from build123d import *

# Parameters (mm, degrees)
EXTRUDE_1_DEPTH          = 22
PATTERN_LINEAR_1_COUNT   = 2
PATTERN_LINEAR_1_PITCH   = 23.5
CUT_EXTRUDE_1_DEPTH      = 38.269290307
CUT_EXTRUDE_1_DEPTH_BACK = 38.269290307
SKETCH_4_W               = 15.894607506
SKETCH_4_H               = 11.25
SKETCH_4_W_2             = 16.409425433
SKETCH_4_H_2             = 14.25
SKETCH_5_R               = 2.5
CUT_EXTRUDE_2_DEPTH      = 45.469793118


with BuildPart() as part:
    # 草图1 → 凸台-拉伸1 (new, symmetric)
    with BuildSketch(Plane.XY):
        with BuildLine():
            Line((29, -5.5), (29, -8))
            Line((29, -8), (1, -8))
            Line((1, -8), (-1.370141735, -7.373785434))
            ThreePointArc((-1.370141735, -7.373785434), (-4.794472702, 5.767411162), (7.5, 0))
            Line((7.5, 0), (25.406366901, 0))
            ThreePointArc((25.406366901, 0), (25.916831332, -0.140101131), (26.284262474, -0.521147869))
            Line((26.284262474, -0.521147869), (29, -5.5))
        make_face()
    extrude(amount=EXTRUDE_1_DEPTH, both=True)

    # 草图3 → 切除-旋转1 (revolve, cut)
    with BuildSketch(Plane.XY.offset(11.75), mode=Mode.PRIVATE) as cut_revolve_1_sk:
        Polygon((24, 0), (17.5, 0), (17.5, -8), (20.75, -8), (20.75, -4), (24, -1), align=None)
    cut_revolve_1 = revolve(cut_revolve_1_sk.sketch.rotate(Axis((17.5, -8, 11.75), (0, 1, 0)), 90), axis=Axis((17.5, -8, 11.75), (0, 1, 0)), mode=Mode.SUBTRACT)

    # 阵列(线性)1: 切除-旋转1 ×2
    with Locations(*[(0, 0, -i * PATTERN_LINEAR_1_PITCH) for i in range(1, PATTERN_LINEAR_1_COUNT)]):
        add(cut_revolve_1, mode=Mode.SUBTRACT)

    # 草图4 → 切除-拉伸1 (cut, two sides: drawn at the far end of the back side and taken through both)
    with BuildSketch(Plane(origin=(0, 0, 0), x_dir=(1, 0, 0), z_dir=(0, 1, 0)).offset(-CUT_EXTRUDE_1_DEPTH_BACK)):
        with Locations((0.004095995, -16.375)):
            Rectangle(SKETCH_4_W, SKETCH_4_H)
        with Locations((0.261504959, 5.625)):
            Rectangle(SKETCH_4_W_2, SKETCH_4_H_2)
    extrude(amount=CUT_EXTRUDE_1_DEPTH + CUT_EXTRUDE_1_DEPTH_BACK, mode=Mode.SUBTRACT)

    # 草图5 → 切除-拉伸2 (cut, through all)
    with BuildSketch(Plane.XY.offset(10.75)):
        Circle(SKETCH_5_R)
    extrude(amount=-CUT_EXTRUDE_2_DEPTH, mode=Mode.SUBTRACT)


solid = part.part
Could you check a few things on this model? Use its own coordinates, in mm. A direction names the side the tool comes from. Give positions to 0.01 mm unless a question says otherwise; leave off trailing zeros. Order: outer loops, then holes, each group sorted by start corner. A loop starts at its lowest first (then second) coordinate and runs counter-clockwise, first axis right, second up. Notation, with made-up numbers: (2.5, -6.75) - (60.5, -6.75) arc R22 cw to (60.5, 13.25) - close; hole circle Ø2 at (62.25, 77). An arc over 180 degrees is marked (long way). One line per question, with ' | ' between items. Start each with the question number.
Item 1: I want a section at D-D on x = -3. Write out the boundary of the cut face in (y, z).
Item 2: I need wall thicknesses on probe 1 along Z at (x, y) = (3.5, 3.75); probe 2 along X at (y, z) = (-0.5, -14); probe 3 along Z at (x, y) = (20.5, -4.25). Which ranges of each line are inside material? Lowest first, please. Write a range as [from, to].
Item 3: For faces 5 (the cylindrical face through (12.019, -0.493, 8.256)), 6 (the flat face through (2, -2, 1.5)), 7 (the flat face through (7, -2, -22)), 8 (the flat face through (2, -2, 10.75)), 9 (the flat face through (15, -8, 0)), which set-ups out of +Z, -Z, +X, -X, +Y, -Y let a thin tool reach every point of the face, with its end or its side?
Item 4: Thinking about a two-plate mould opening in X: for faces 1 (the cylindrical face through (14.278, -5.972, 12.173)), 2 (the flat face through (-0.17, -7.69, 6.19)), 3 (the cylindrical face through (-4.975, 5.613, 6.19)), 4 (the cylindrical face through (-0.54, -2.44, 6.19)), which applies, pulls with the +X half, pulls with the -X half, needs draft (parallel to the pull), parting line crosses it, or undercut?
Item 5: I'm going to push flat-ended pins straight in: pin 1 Ø6.5 at (x, y) = (0, 0) entering from +Z; pin 2 Ø4 at (y, z) = (-5, 15.5) entering from -X; pin 3 Ø6 at (y, z) = (0, -8.5) entering from -X; pin 4 Ø1.5 at (y, z) = (1.5, 17) entering from -X. Where does each tip first touch, or does it pass through?
Item 6: I want a section at A-A on y = -2. Write out the boundary of the cut face in (x, z), then the cut area to 3 significant figures.
Item 7: I want a section at C-C on x = 17.5. Write out the boundary of the cut face in (y, z).
Item 8: I want a section at B-B on z = -11.75. Write out the boundary of the cut face in (x, y).
Verdict:
1) outline: (-6.87, -22) - (6.87, -22) - (6.87, -12.75) - (-6.87, -12.75) - close; (-6.87, 1.5) - (6.87, 1.5) - (6.87, 10.75) - (-6.87, 10.75) - close
2) probe 1: [-22, -12.75], [1.5, 10.75] | probe 2: [-7.48, -2.45], [2.45, 11.4], [23.6, 26.27] | probe 3: [-22, -13], [-10.5, 10.5], [13, 22]
3) face 5: +Y | face 6: -X, +Y, -Y | face 7: -Z, +X, -X, +Y, -Y | face 8: +Z, -X, +Y, -Y | face 9: +Z, -Z, +X, -X, -Y
4) face 1: undercut | face 2: pulls with the -X half | face 3: parting line crosses it | face 4: undercut
5) pin 1: z = 10.75 | pin 2: x = 7.95 | pin 3: x = 8.47 | pin 4: through
6) outline: (-7.23, -22) - (-1.5, -22) - (-1.5, -12.75) - (-7.23, -12.75) - close; (-7.23, 1.5) - (-1.5, 1.5) - (-1.5, 10.75) - (-7.23, 10.75) - close; (1.5, -22) - (27.09, -22) - (27.09, 22) - (7.95, 22) - (7.95, 10.75) - (1.5, 10.75) - (1.5, 1.5) - (8.47, 1.5) - (8.47, -12.75) - (1.5, -12.75) - close; hole circle Ø10.83 at (17.5, -11.75); hole circle Ø10.83 at (17.5, 11.75) | area: 876 mm^2
7) outline: (-8, -22) - (0, -22) - (0, -18.25) - (-1, -18.25) - (-4, -15) - (-8, -15) - close; (-8, -8.5) - (-4, -8.5) - (-1, -5.25) - (0, -5.25) - (0, 5.25) - (-1, 5.25) - (-4, 8.5) - (-8, 8.5) - close; (-8, 15) - (-4, 15) - (-1, 18.25) - (0, 18.25) - (0, 22) - (-8, 22) - close
8) outline: (8.47, -8) - (14.25, -8) - (14.25, -4) - (11, -1) - (11, 0) - (8.47, 0) - close; (20.75, -8) - (29, -8) - (29, -5.5) - (26.28, -0.52) arc R1 ccw to (25.41, 0) - (24, 0) - (24, -1) - (20.75, -4) - close
